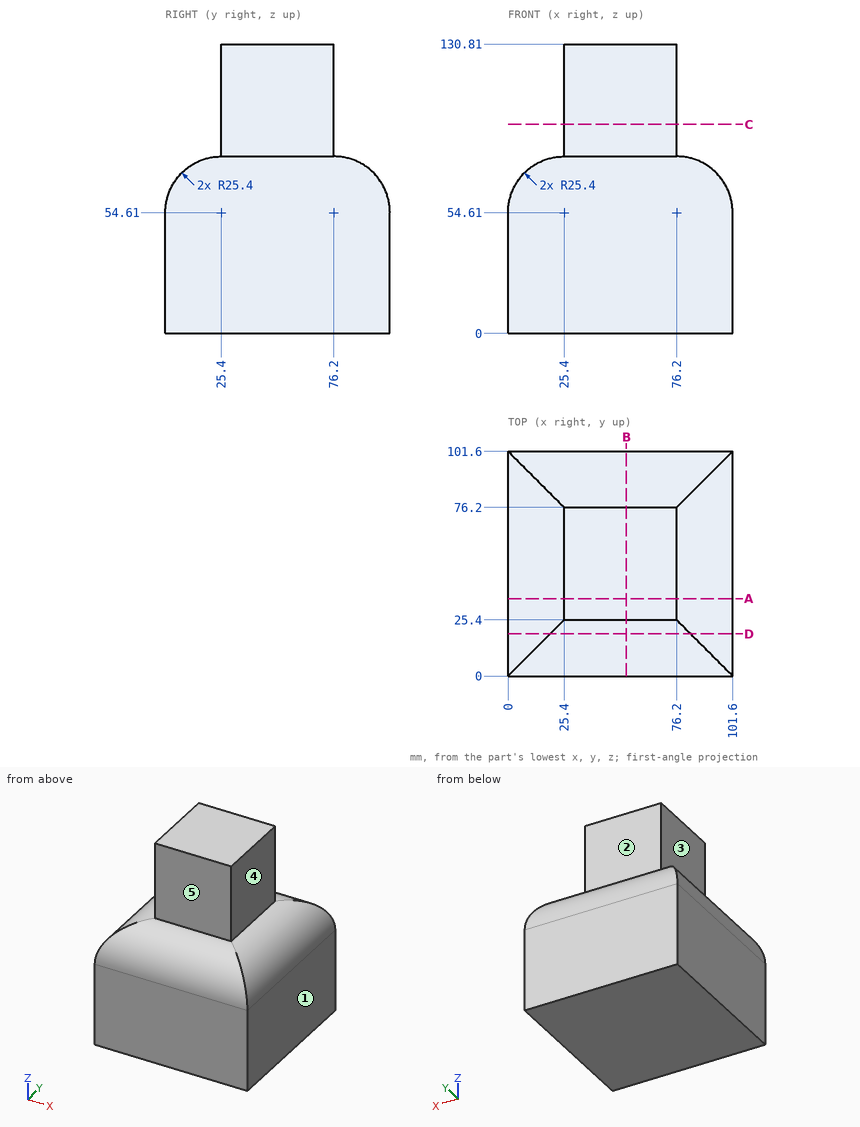
Geometry: see drawing. Coordinates: mm, zero at the bounding-box minimum. A direction names the side the tool comes from. Coordinates: 2 decimals unless noted, no trailing zeros. Write each loop counter-clockwise with the first axis right and the second up, starting at its lowest first coordinate (ties: lowest second). Pieces come first, ordered by that corner, then holes.
1) Set-up query: the marked faces 1, 2, 3, 4 and 5. Return all of +Z, -Z, +X, -X, +Y, -Y with unobstructed straight access to the full face (end or side cutting, diameter ignored); none if empty.
2) Section A-A on y = 35. Output: boundary loops of the cut face in (x, z).
3) Material intervals for line 1 along Y through (x, z) = (66, 105); line 2 along Z through (x, y) = (17.5, 65), sorted ascending.
4) Pin query (flat end, axial travel): pin 1 Ø4 at (y, z) = (78.5, 61) entering from -X; pin 2 Ø4 at (y, z) = (24, 72) entering from -X; pin 3 Ø8 at (y, z) = (23.5, 108.5) entering from -X. Return the tip coordinate at first contact, or that it passes through.
5) Section C-C on z = 94.5. Output: boundary loops of the cut face in (x, y), and give its area (3 significant figures).
6) Section D-D on y = 19. Output: boundary loops of the cut face in (x, z).
Check result:
1. face 1: +Z, -Z, +X, +Y, -Y
1. face 2: +Z, +X, -X, +Y
1. face 3: +Z, -X, +Y, -Y
1. face 4: +Z, +X, +Y, -Y
1. face 5: +Z, +X, -X, -Y
2. outline: (0, 0) - (101.6, 0) - (101.6, 54.61) arc R25.4 ccw to (76.2, 80.01) - (76.2, 130.81) - (25.4, 130.81) - (25.4, 80.01) arc R25.4 ccw to (0, 54.61) - close
3. line 1: y = 25.4 to 76.2
3. line 2: z = 0 to 78.75
4. pin 1: stops at x = 0.38
4. pin 2: stops at x = 5.19
4. pin 3: stops at x = 25.4
5. outline: (25.4, 25.4) - (76.2, 25.4) - (76.2, 76.2) - (25.4, 76.2) - close
5. area: 2,580 mm2
6. outline: (0, 0) - (101.6, 0) - (101.6, 54.61) arc R25.4 ccw to (82.6, 79.19) - (19, 79.19) arc R25.4 ccw to (0, 54.61) - close
